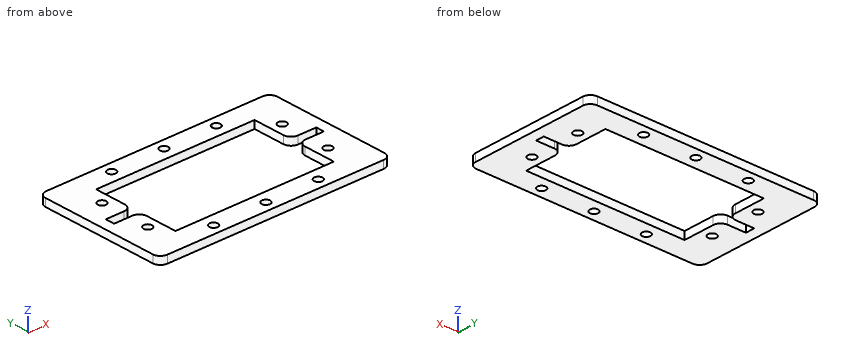
```python
from build123d import *

# Parameters (mm, degrees)
F0_R     = 2.75
F1_DEPTH = 5


with BuildPart() as f1:
    # F0 (on Top) → F1 (new body)
    with BuildSketch(Plane.XY):
        with BuildLine():
            Line((0, 25.5), (0, 0))
            Line((0, 0), (14, 0))
            Line((14, 0), (14, 20.5))
            ThreePointArc((14, 20.5), (12.5355339059, 24.0355339059), (9, 25.5))
            Line((9, 25.5), (0, 25.5))
        make_face()
        with Locations((6.85, 12.05)):
            Circle(F0_R, mode=Mode.SUBTRACT)
        with BuildLine():
            Line((14, 0), (0, 0))
            Line((0, 0), (-10, 0))
            Line((-10, 0), (-10, -10))
            ThreePointArc((-10, -10), (-8.5355339059, -13.5355339059), (-5, -15))
            Line((-5, -15), (0, -15))
            Line((0, -15), (132, -15))
            Line((132, -15), (132, 0))
            Line((132, 0), (118, 0))
            Line((118, 0), (14, 0))
        make_face()
        with Locations((31.625, -8.15)):
            Circle(F0_R, mode=Mode.SUBTRACT)
        with Locations((66, -8.15)):
            Circle(F0_R, mode=Mode.SUBTRACT)
        with Locations((100.375, -8.15)):
            Circle(F0_R, mode=Mode.SUBTRACT)
        Polygon((-10, 0), (0, 0), (0, 25.5), (-3, 25.5), (-3, 28.5), (-3, 31.5), (0, 31.5), (0, 57), (-10, 57), align=None)
        with BuildLine():
            Line((118, 20.75), (118, 0))
            Line((118, 0), (132, 0))
            Line((132, 0), (132, 25.75))
            Line((132, 25.75), (123, 25.75))
            ThreePointArc((123, 25.75), (119.4644660941, 24.2855339059), (118, 20.75))
        make_face()
        with Locations((125.15, 12.05)):
            Circle(F0_R, mode=Mode.SUBTRACT)
        with BuildLine():
            Line((-10, 67), (-10, 57))
            Line((-10, 57), (0, 57))
            Line((0, 57), (0, 72))
            Line((0, 72), (-5, 72))
            ThreePointArc((-5, 72), (-8.5355339059, 70.5355339059), (-10, 67))
        make_face()
        with BuildLine():
            Line((0, 57), (0, 31.5))
            Line((0, 31.5), (9, 31.5))
            ThreePointArc((9, 31.5), (12.5355339059, 32.9644660941), (14, 36.5))
            Line((14, 36.5), (14, 57))
            Line((14, 57), (0, 57))
        make_face()
        with Locations((6.85, 44.95)):
            Circle(F0_R, mode=Mode.SUBTRACT)
        with BuildLine():
            Line((142, 0), (132, 0))
            Line((132, 0), (132, -15))
            Line((132, -15), (137, -15))
            ThreePointArc((137, -15), (140.5355339059, -13.5355339059), (142, -10))
            Line((142, -10), (142, 0))
        make_face()
        Polygon((132, 25.75), (132, 0), (142, 0), (142, 57), (132, 57), (132, 31.25), (135, 31.25), (135, 28.25), (135, 25.75), align=None)
        Polygon((0, 72), (0, 57), (14, 57), (118, 57), (132, 57), (132, 72), (100.375, 72), align=None)
        with Locations((31.625, 65.15)):
            Circle(F0_R, mode=Mode.SUBTRACT)
        with Locations((66, 65.15)):
            Circle(F0_R, mode=Mode.SUBTRACT)
        with BuildLine():
            ThreePointArc((103.125, 65.15), (98.4304563517, 63.2054563517), (100.375, 67.9))
            ThreePointArc((100.375, 67.9), (102.3195436483, 67.0945436483), (103.125, 65.15))
        make_face(mode=Mode.SUBTRACT)
        with BuildLine():
            Line((123, 31.25), (132, 31.25))
            Line((132, 31.25), (132, 57))
            Line((132, 57), (118, 57))
            Line((118, 57), (118, 36.25))
            ThreePointArc((118, 36.25), (119.4644660941, 32.7144660941), (123, 31.25))
        make_face()
        with Locations((125.15, 44.95)):
            Circle(F0_R, mode=Mode.SUBTRACT)
        with BuildLine():
            Line((132, 57), (142, 57))
            Line((142, 57), (142, 67))
            ThreePointArc((142, 67), (140.5355339059, 70.5355339059), (137, 72))
            Line((137, 72), (132, 72))
            Line((132, 72), (132, 57))
        make_face()
    extrude(amount=F1_DEPTH)


solid = f1.part
```
Verification items for the finished model (mm, model axes). Round coordinates to 2 decimals unless told otherwise and drop trailing zeros. Order: outer loops, then holes, each group sorted by start corner. A loop starts at its lowest first (then second) coordinate and runs counter-clockwise, first axis right, second up. Notation, with made-up numbers: (55, 49) -> (77, 49) arc R24 cw to (77, 70) -> close; hole circle Ø9 at (81.5, 36.5). An arc over 180 degrees is marked (long way). Put each result on its own line as item: value. Start each with the question number.
(1) Depth check by flat-ended pin: pin 1 Ø3.5 at (x, y) = (100.375, -8.15) entering from +Z; pin 2 Ø6.5 at (x, y) = (31.625, 65.15) entering from +Z. Enter the tip coordinate at first touch or a pass-through.
(2) Section check C-C (x = 56). Enter the section's corners in (y, z), then the cut area to 3 significant figures.
(3) Section check B-B (y = 52.5). Enter the section's corners in (x, z), then the cut area to 3 significant figures.
(4) Material ranges on line 1 along X through (y, z) = (45, 0.6); line 2 along Y through (x, z) = (125.5, 3.2); line 3 along Y through (x, z) = (6.85, 1), recorded low to high.
(5) Section check A-A (x = 125.15). Enter the section's corners in (y, z).
(6) Section check D-D (y = 12.05). Enter the section's corners in (x, z).
Completed:
1. pin 1: passes through
1. pin 2: stops at z = 5
2. outline: (-15, 0) -> (0, 0) -> (0, 5) -> (-15, 5) -> close; (57, 0) -> (72, 0) -> (72, 5) -> (57, 5) -> close
2. area: 150 mm2
3. outline: (-10, 0) -> (14, 0) -> (14, 5) -> (-10, 5) -> close; (118, 0) -> (142, 0) -> (142, 5) -> (118, 5) -> close
3. area: 240 mm2
4. line 1: x = -10 to 4.1, 9.6 to 14, 118 to 122.4, 127.9 to 142
4. line 2: y = -15 to 9.32, 14.78 to 25.75, 31.25 to 42.22, 47.68 to 72
4. line 3: y = -15 to 9.3, 14.8 to 25.5, 31.5 to 42.2, 47.7 to 72
5. outline: (-15, 0) -> (9.3, 0) -> (9.3, 5) -> (-15, 5) -> close; (14.8, 0) -> (25.75, 0) -> (25.75, 5) -> (14.8, 5) -> close; (31.25, 0) -> (42.2, 0) -> (42.2, 5) -> (31.25, 5) -> close; (47.7, 0) -> (72, 0) -> (72, 5) -> (47.7, 5) -> close
6. outline: (-10, 0) -> (4.1, 0) -> (4.1, 5) -> (-10, 5) -> close; (9.6, 0) -> (14, 0) -> (14, 5) -> (9.6, 5) -> close; (118, 0) -> (122.4, 0) -> (122.4, 5) -> (118, 5) -> close; (127.9, 0) -> (142, 0) -> (142, 5) -> (127.9, 5) -> close
